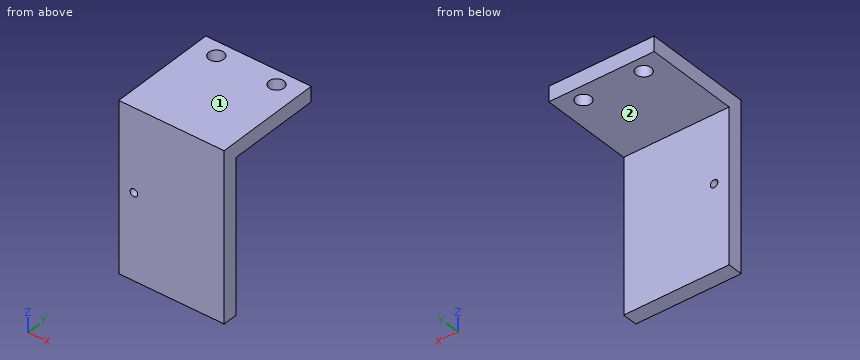
```python
from build123d import *

# Parameters (mm, degrees)
SKETCH1_R           = 2.5
BOSS_EXTRUDE1_DEPTH = 5
SKETCH2_W           = 35
SKETCH2_H           = 55.8
SKETCH2_R           = 1.25
BOSS_EXTRUDE2_DEPTH = 5


with BuildPart() as part:
    # Sketch1 → Boss-Extrude1 (new body)
    with BuildSketch(Plane.XY):
        Polygon((-17.5, 5), (17.5, 5), (17.5, -5), (17.5, -26), (-17.5, -26), (-17.5, -5), align=None)
        with Locations((-10, 0)):
            Circle(SKETCH1_R, mode=Mode.SUBTRACT)
        with Locations((10, 0)):
            Circle(SKETCH1_R, mode=Mode.SUBTRACT)
    extrude(amount=BOSS_EXTRUDE1_DEPTH)

    # Sketch2 → Boss-Extrude2 (add)
    with BuildSketch(Plane.XZ.offset(26)):
        with Locations((0, -22.9)):
            Rectangle(SKETCH2_W, SKETCH2_H)
        with Locations((-12.5, -22.4)):
            Circle(SKETCH2_R, mode=Mode.SUBTRACT)
    extrude(amount=BOSS_EXTRUDE2_DEPTH)


solid = part.part
```
Here's how the part is built. I have some questions about the finished solid (model axes, mm). Face numbers are marked on the shaded views. A direction names the side the tool comes from. Coordinates: 2 decimals unless noted, no trailing zeros. Loops run counter-clockwise (first coordinate to the right, second up) from the corner with the lowest first, then second, coordinate; pieces in that order, holes last. Notation, with made-up numbers: (72, 75.5) - (103, 75.5) arc R9 cw to (103, 92.5) - close; hole circle Ø7 at (22, 80). An arc over 180 degrees is marked (long way). Return JSON: item names as keys, results as strings. Group by question number.
Item 1: If we section it at A-A on x = 8.5: Write out the boundary of the cut face in (y, z), and give its area (3 significant figures).
Item 2: If we section it at B-B on z = -22.4: Write out the boundary of the cut face in (x, y), and give its area (4 significant figures).
Item 3: Will these pins go through, and if not, where does the flat tip stop? P1, Ø10.5, axis at x = -2, z = -31, coming from the +Y side; P2, Ø5, axis at x = -4, y = -14, coming from the -Z side; P3, Ø1.5, axis at x = -12.5, z = -22.4, coming from the -Y side.
Item 4: I need wall thicknesses on line 1 (Y direction, x = 10, z = 3); line 2 (Z direction, x = -15, y = -25.5); line 3 (Z direction, x = -12.5, y = -28.55). Which ranges of each line are inside material? Lowest first, please. Write a range as from..to.
Item 5: If we section it at D-D on x = -10: Write out the boundary of the cut face in (y, z).
Item 6: On a 3-axis mill with a long thin cutter (end or side, diameter ignored), from which of +Z, -Z, +X, -X, +Y, -Y can I reach the whole of each face in a straight line? I mean the marked faces 1 and 2. Say none if no direction works.
Item 7: If we section it at C-C on y = 0: Write out the boundary of the cut face in (x, z).
Calculated:
{
 "1": {"outline": "(-31, -50.8) - (-26, -50.8) - (-26, 0) - (-2, 0) - (-2, 5) - (-31, 5) - close; (2, 0) - (5, 0) - (5, 5) - (2, 5) - close", "area": "414 mm^2"},
 "2": {"outline": "(-17.5, -31) - (-13.75, -31) - (-13.75, -26) - (-17.5, -26) - close; (-11.25, -31) - (17.5, -31) - (17.5, -26) - (-11.25, -26) - close", "area": "162.5 mm^2"},
 "3": {"P1": "stops at y = -26", "P2": "stops at z = 0", "P3": "passes through"},
 "4": {"line 1": "y = -31..-2.5, 2.5..5", "line 2": "z = 0..5", "line 3": "z = -50.8..-23.65, -21.15..5"},
 "5": {"outline": "(-31, -50.8) - (-26, -50.8) - (-26, 0) - (-2.5, 0) - (-2.5, 5) - (-31, 5) - close; (2.5, 0) - (5, 0) - (5, 5) - (2.5, 5) - close"},
 "6": {"face 1": "+Z, +X, -X, +Y, -Y", "face 2": "-Z, +X, -X, +Y"},
 "7": {"outline": "(-17.5, 0) - (-12.5, 0) - (-12.5, 5) - (-17.5, 5) - close; (-7.5, 0) - (7.5, 0) - (7.5, 5) - (-7.5, 5) - close; (12.5, 0) - (17.5, 0) - (17.5, 5) - (12.5, 5) - close"}
}
